Can you work these out from the model? Positions are in its coordinate system, mm. Give positions to 0.01 mm unless a question says otherwise; leave off trailing zeros. Loops run counter-clockwise (first coordinate to the right, second up) from the corner with the lowest first, then second, coordinate; pieces in that order, holes last. Notation, with made-up numbers: M 39.5,82.5 L 75.5,82.5 A23 ccw 75.5,93.5 Z; hole C -7,84 d8. An arc over 180 degrees is marked long. Put each result on its own line as item: value. Start each with the question number.
1) Imagine slicing it at A-A (y = 1.55). Write out the boundary of the cut face in (x, z).
2) Please list where these lines run through material, in increasing order: line 1 along Z through (x, y) = (-1.5, 1.05); line 2 along X through (y, z) = (1.35, 0.25); line 3 along X through (y, z) = (2.45, -1.25). Write a range as from..to.
3) For P1, Ø2, axis at x = 0, z = 0, coming from the -Y side; P2, Ø1, axis at y = 1.5, z = -1.5, coming from the +X side, each with a flat end and sliding along its axis, tell me the tip position at first contact or that it passes through.
from build123d import *

# Parameters (mm, degrees)
BOSS_EXTRUDE1_DEPTH = 3.2
M4_TAPPED_HOLE1_D   = 3.3


with BuildPart() as part:
    # Sketch1 → Boss-Extrude1 (new body)
    with BuildSketch(Plane(origin=(0, 0, 0), x_dir=(1, 0, 0), z_dir=(0, 1, 0))):
        Polygon((-2.020725942, -3.5), (2.020725942, -3.5), (4.041451884, 0), (2.020725942, 3.5), (-2.020725942, 3.5), (-4.041451884, 0), align=None)
    extrude(amount=BOSS_EXTRUDE1_DEPTH)

    # Sketch2 → Cut-Revolve1 (revolve, cut)
    with BuildSketch(Plane(origin=(0, 0, 0), x_dir=(0, 0, -1), z_dir=(1, 0, 0))):
        Polygon((5.627238375, 1.228161648), (3.5, 0), (5.627238375, 0), align=None)
        Polygon((3.5, 3.2), (5.644714185, 3.2), (5.644714185, 1.961748688), align=None)
    revolve(axis=Axis((0, 0, 0), (0, 1, 0)), mode=Mode.SUBTRACT)

    # M4 Tapped Hole1 (through all)
    with Locations(Plane.ZX.offset(3.2)):
        with Locations((0, 0)):
            Hole(M4_TAPPED_HOLE1_D / 2)


solid = part.part
Recorded:
1. outline: M -4.04,0 L -2.02,-3.5 L 2.02,-3.5 L 4.04,0 L 2.02,3.5 L -2.02,3.5 Z; hole C 0,0 d3.3
2. line 1: -3.5..-0.69, 0.69..3.5
2. line 2: -3.9..-1.63, 1.63..3.9
2. line 3: -3.32..-1.08, 1.08..3.32
3. P1: through
3. P2: x = 3.46
